Autodesk Inventor part; units mm, degrees
ref_plane "YZ Plane" through (0, 0, 0) normal (1, 0, 0) x (0, 1, 0)
ref_plane "XZ Plane" through (0, 0, 0) normal (0, 1, 0) x (-1, 0, 0)
ref_plane "XY Plane" through (0, 0, 0) normal (0, 0, 1) x (1, 0, 0)
sketch "Sketch1" plane through (0, 0, 0) normal (0, 0, 1) x (1, 0, 0)
  line L0 (0, 0) -> (-482.6, 0)
  line L1 (-482.6, 0) -> (-482.6, 44)
  line L2 (-482.6, 44) -> (0, 44)
  line L3 (0, 44) -> (0, 0)
  arc A0 (-473.8, 41.375) -> (-473.8, 34.375) centre (-473.8, 37.875) ccw
  arc A1 (-473.8, 9.625) -> (-473.8, 2.625) centre (-473.8, 6.125) ccw
  arc A2 (-8.8, 34.375) -> (-8.8, 41.375) centre (-8.8, 37.875) ccw
  arc A3 (-8.8, 2.625) -> (-8.8, 9.625) centre (-8.8, 6.125) ccw
  line L4 (-473.8, 41.375) -> (-470.8, 41.375)
  line L5 (-473.8, 34.375) -> (-470.8, 34.375)
  arc A4 (-470.8, 34.375) -> (-470.8, 41.375) centre (-470.8, 37.875) ccw
  line L6 (-8.8, 41.375) -> (-11.8, 41.375)
  line L7 (-8.8, 34.375) -> (-11.8, 34.375)
  arc A5 (-11.8, 41.375) -> (-11.8, 34.375) centre (-11.8, 37.875) ccw
  line L8 (-8.8, 9.625) -> (-11.8, 9.625)
  line L9 (-8.8, 2.625) -> (-11.8, 2.625)
  arc A6 (-11.8, 9.625) -> (-11.8, 2.625) centre (-11.8, 6.125) ccw
  line L10 (-473.8, 9.625) -> (-470.8, 9.625)
  line L11 (-473.8, 2.625) -> (-470.8, 2.625)
  arc A7 (-470.8, 2.625) -> (-470.8, 9.625) centre (-470.8, 6.125) ccw
  dimension "d0" = 44
  dimension "d1" = 482.6
  dimension "d5" = 31.75
  dimension "d6" = 7
  dimension "d8" = 31.75
  dimension "d9" = 465
  dimension "d10" = 465
  dimension "d11" = 8.8
  dimension "d12" = 8.8
  dimension "d13" = 6.125
  dimension "d14" = 6.125
  dimension "d15" = 6.125
  dimension "d16" = 8.8
  dimension "d17" = 8.8
  dimension "d18" = 6.125
  dimension "d43" = 3
  dimension "d45" = 3.5
extrude "Frame" add sketch "Sketch1" along normal blind 3
sketch "Sketch2" plane through (0, 0, 3) normal (0, 0, 1) x (1, 0, 0)
  line L0 (-30, 4) -> (-170, 4)
  line L1 (-170, 4) -> (-170, 40)
  line L2 (-170, 40) -> (-30, 40)
  line L3 (-30, 40) -> (-30, 4)
  line L4 (-452.6003, 40) -> (-312.6003, 40)
  line L5 (-312.6003, 40) -> (-312.6003, 4)
  line L6 (-312.6003, 4) -> (-452.6003, 4)
  line L7 (-452.6003, 4) -> (-452.6003, 40)
  line L8 (0, 0) -> (0, 44)
  line L9 (0, 44) -> (-482.6, 44)
  line L10 (-482.6, 44) -> (-482.6, 0)
  point P0 (-30, 22)
  point P1 (-312.6003, 22)
  dimension "d21" = 140
  dimension "d22" = 36
  dimension "d25" = 30
  dimension "d26" = 22
  dimension "d27" = 22
  dimension "d28" = 29.9997
extrude "PI_Holes" cut sketch "Sketch2" against normal blind 5
sketch "Sketch4" plane through (0, 0, 3) normal (0, 0, 1) x (1, 0, 0)
  circle A0 centre (-26, 22) radius 2
  circle A1 centre (-174, 22) radius 2
  circle A2 centre (-308.6003, 22) radius 2
  circle A3 centre (-456.6003, 22) radius 2
  circle A4 centre (-456.6003, 22) radius 2.25
  circle A5 centre (-308.6003, 22) radius 2.25
  circle A6 centre (-174, 22) radius 2.25
  circle A7 centre (-26, 22) radius 2.25
  point P0 (0, 0)
  dimension "d35" = 4
  dimension "d36" = 4.5
  dimension "d37" = 4.5
  dimension "d38" = 4.5
  dimension "d39" = 4.5
extrude "Mounting_Holes" cut sketch "Sketch4" against normal through all contours A0 | A1 | A2 | A3 | A4 | A5 | A6 | A7
properties part number "WoodPanel" material "Wood (Walnut)"
Geometry check sheet. Reference: the model listing, model coordinates, mm. Coordinates: 2 decimals unless noted, no trailing zeros. Loops run counter-clockwise (first coordinate to the right, second up) from the corner with the lowest first, then second, coordinate; pieces in that order, holes last. Notation, with made-up numbers: (4.5, 86) -> (12.5, 86) arc R17 cw to (12.5, 114) -> close; hole circle Ø9 at (79, 36.5). An arc over 180 degrees is marked (long way). Put each result on its own line as item: value.
1) Cross-section at A-A on z = 1.4. Count the separate pieces of the cut face and the enclosed holes in it, plus the area to 3 significant figures.
Result set:
separate pieces: 1
enclosed holes: 10
area: 10,900 mm^2
2) Cross-section at B-B on x = -369. Record the boundary of the cut face in (y, z), plus the area to 3 significant figures.
Result set:
outline: (0, 0) -> (4, 0) -> (4, 3) -> (0, 3) -> close; (40, 0) -> (44, 0) -> (44, 3) -> (40, 3) -> close
area: 24.0 mm^2
3) Thickness scan on line 1 (X direction, y = 15.5, z = 1.95); line 2 (X direction, y = 6, z = 2.65); line 3 (Y direction, x = -26, z = 1.05). Record the ranges inside material, lowest first.
Result set:
line 1: x = -482.6 to -452.6, -312.6 to -170, -30 to 0
line 2: x = -482.6 to -477.3, -467.3 to -452.6, -312.6 to -170, -30 to -15.3, -5.3 to 0
line 3: y = 0 to 19.75, 24.25 to 44
